from build123d import *

# Parameters (mm, degrees)
SKETCH3_OUTSIDE_W  = 93.666
SKETCH3_OUTSIDE_H  = 93.666
SKETCH3_OUTSIDE_R  = 6.5
CUT_EXTRUDE1_DEPTH = 21
SKETCH4_W          = 2.5
SKETCH4_H          = 24.819260196
SKETCH7_W          = 2.358889098
SKETCH7_H          = 15
CUT_EXTRUDE2_DEPTH = 12
CIRPATTERN1_COUNT  = 2
CIRPATTERN1_ANGLE  = 180
CHAMFER1_SIZE      = 0.5


with BuildPart() as part:
    # Sketch1 → Revolve1 (revolve)
    with BuildSketch(Plane(origin=(0, 0, 0), x_dir=(0, 0, -1), z_dir=(1, 0, 0)), mode=Mode.PRIVATE) as revolve1_sk:
        Polygon((14, 13), (0.5, 13), (0, 12.5), (0, 7.95), (2, 5.95), (19, 5.95), (20.171678207, 4), (38, 4), (40.403442476, 0), (44, 0), (44, 9.45), (43.5, 9.95), (41.5, 9.95), (41.5, 8.15), (38.3, 8.15), (38.3, 9.95), (35.8, 9.95), (35.8, 8.15), (30.8, 8.15), (30.8, 9.95), (28.3, 9.95), (28.3, 8.15), (25.1, 8.15), (25.1, 9.95), (21, 9.95), (21, 35), (14, 35), align=None)
    revolve(revolve1_sk.sketch.rotate(Axis((0, 0, 0), (0, 0, -1)), 90), axis=Axis((0, 0, 0), (0, 0, -1)))

    # Sketch3 outside → Cut-Extrude1 (cut)
    # profile 1 of 3: a face of its own
    with BuildSketch(Plane.XY):
        Rectangle(SKETCH3_OUTSIDE_W, SKETCH3_OUTSIDE_H)
        with BuildLine():
            Line((-20, 11.295529415), (-20, -11.295529415))
            ThreePointArc((-20, -11.295529415), (-19.765527652, -13.448311261), (-19.073106065, -15.500139543))
            Line((-19.073106065, -15.500139543), (-13.185668477, -28.204610128))
            ThreePointArc((-13.185668477, -28.204610128), (-9.495586596, -32.427517466), (-4.112562412, -34))
            Line((-4.112562412, -34), (4.112562412, -34))
            ThreePointArc((4.112562412, -34), (9.495586596, -32.427517466), (13.185668477, -28.204610128))
            Line((13.185668477, -28.204610128), (19.073106065, -15.500139543))
            ThreePointArc((19.073106065, -15.500139543), (19.765527652, -13.448311261), (20, -11.295529415))
            Line((20, -11.295529415), (20, 11.295529415))
            ThreePointArc((20, 11.295529415), (19.765527652, 13.448311261), (19.073106065, 15.500139543))
            Line((19.073106065, 15.500139543), (13.185668477, 28.204610128))
            ThreePointArc((13.185668477, 28.204610128), (9.495586596, 32.427517466), (4.112562412, 34))
            Line((4.112562412, 34), (-4.112562412, 34))
            ThreePointArc((-4.112562412, 34), (-9.495586596, 32.427517466), (-13.185668477, 28.204610128))
            Line((-13.185668477, 28.204610128), (-19.073106065, 15.500139543))
            ThreePointArc((-19.073106065, 15.500139543), (-19.765527652, 13.448311261), (-20, 11.295529415))
        make_face(mode=Mode.SUBTRACT)
    # profile 2 of 3: a face of its own
    with BuildSketch(Plane.XY):
        with Locations((0, 24)):
            Circle(SKETCH3_OUTSIDE_R)
    # profile 3 of 3: a face of its own
    with BuildSketch(Plane.XY):
        with Locations((0, -24)):
            Circle(SKETCH3_OUTSIDE_R)
    extrude(amount=-CUT_EXTRUDE1_DEPTH, mode=Mode.SUBTRACT)

    # Sketch4 → Cut-Revolve1 (revolve, cut)
    with BuildSketch(Plane(origin=(0, 0, 0), x_dir=(0, 0, -1), z_dir=(1, 0, 0)), mode=Mode.PRIVATE) as cut_revolve1_sk:
        with Locations((34.55, 0)):
            Rectangle(SKETCH4_W, SKETCH4_H)
    revolve(cut_revolve1_sk.sketch.rotate(Axis((0, 12.409630098, -33.3), (0, -1, 0)), 180), axis=Axis((0, 12.409630098, -33.3), (0, -1, 0)), mode=Mode.SUBTRACT)

    # Sketch7 → Cut-Extrude2 (cut)
    with BuildSketch(Plane.XY):
        with Locations((-13.179444549, -0.815585695)):
            Rectangle(SKETCH7_W, SKETCH7_H)
    cut_extrude2 = extrude(amount=-CUT_EXTRUDE2_DEPTH, mode=Mode.SUBTRACT)

    # CirPattern1: Cut-Extrude2 ×2 about axis
    cirpattern1_axis = Axis((0, 0, 0), (0, 0, 1))
    for i in range(1, CIRPATTERN1_COUNT):
        add(cut_extrude2.rotate(cirpattern1_axis, i * CIRPATTERN1_ANGLE / (CIRPATTERN1_COUNT - 1)), mode=Mode.SUBTRACT)

    # Chamfer1
    chamfer1_edges = [part.edges().sort_by_distance(p)[0] for p in [
        (-6.5, 24, -21),
        (-6.5, 24, -14),
        (-6.5, -24, -21),
        (-6.5, -24, -14),
        (0, 34, -21),
        (-9.495586596, 32.427517466, -21),
        (-16.129387271, 21.852374836, -21),
        (-19.765527652, 13.448311261, -21),
        (-20, 0, -21),
        (-19.765527652, -13.448311261, -21),
        (-16.129387271, -21.852374836, -21),
        (-9.495586596, -32.427517466, -21),
        (0, -34, -21),
        (9.495586596, -32.427517466, -21),
        (16.129387271, -21.852374836, -21),
        (19.765527652, -13.448311261, -21),
        (20, 0, -21),
        (19.765527652, 13.448311261, -21),
        (16.129387271, 21.852374836, -21),
        (9.495586596, 32.427517466, -21),
        (-9.495586596, 32.427517466, -14),
        (0, 34, -14),
        (9.495586596, 32.427517466, -14),
        (16.129387271, 21.852374836, -14),
        (19.765527652, 13.448311261, -14),
        (20, 0, -14),
        (19.765527652, -13.448311261, -14),
        (16.129387271, -21.852374836, -14),
        (9.495586596, -32.427517466, -14),
        (0, -34, -14),
        (-9.495586596, -32.427517466, -14),
        (-16.129387271, -21.852374836, -14),
        (-19.765527652, -13.448311261, -14),
        (-20, 0, -14),
        (-19.765527652, 13.448311261, -14),
        (-16.129387271, 21.852374836, -14),
    ]]
    chamfer(chamfer1_edges, length=CHAMFER1_SIZE)


solid = part.part
CAD build for the part. Positions are in the model's coordinates, mm. A direction names the side the tool comes from. Round coordinates to 2 decimals unless told otherwise and drop trailing zeros. Loops run counter-clockwise (first coordinate to the right, second up) from the corner with the lowest first, then second, coordinate; pieces in that order, holes last. Notation, with made-up numbers: (81, -15.5) - (115, -15.5) arc R10 cw to (115, 1.5) - close; hole circle Ø4 at (72, 49.5). An arc over 180 degrees is marked (long way). Put each result on its own line as item: value.
1. Slice it at C-C on y = -24. List the corners of the cut face in (x, z), and give its area (3 significant figures).
Geometry check:
outline: (-15.13, -20.5) - (-14.58, -21) - (-7, -21) - (-6.5, -20.5) - (-6.5, -14.5) - (-7, -14) - (-14.58, -14) - (-15.13, -14.5) - close; (6.5, -20.5) - (7, -21) - (14.58, -21) - (15.13, -20.5) - (15.13, -14.5) - (14.58, -14) - (7, -14) - (6.5, -14.5) - close
area: 120 mm²
2. Two-plate mould, pull along Z, no slides. Class faces 1 (the conical face through (-9.235, 32.161, -20.865)), 2 (the flat face through (0, 34, -17)), 3 (the flat face through (-15.86, 21.84, -14.25)), 4 (the flat face through (-8.2, -1.5, -28.3)): released by +Z, released by -Z, zero draft, split by the parting line, or undercut.
Geometry check:
face 1: released by -Z
face 2: zero draft
face 3: released by +Z
face 4: undercut
3. Pin check, flat tips, straight feed: P1, Ø21, axis at x = 0, y = -24, coming from the +Z side; P2, Ø4, axis at x = -8.5, z = -20.5, coming from the +Y side; P3, Ø8, axis at x = 13.5, z = -8, coming from the +Y side; P4, Ø1, axis at x = -9.5, z = -26.5, coming from the +Y side. Stop position of each tip, or through.
Geometry check:
P1: z = -14
P2: y = 33.71
P3: y = 8.87
P4: through
4. 3-axis set-ups, long thin cutter, end or side, ignore diameter. For faces 5 (the cylindrical face through (-7.9, 6.05, -29.53)), 6 (the cylindrical face through (-4.385, -4.021, -10.619)), 7 (the flat face through (8.2, -1.5, -25.1)): which of +Z, -Z, +X, -X, +Y, -Y reach the whole face in a straight line?
Geometry check:
face 5: -Z
face 6: +Z
face 7: none
5. Slice it at B-B on z = -5.5. List the corners of the cut face in (x, y), and give its area (3 significant figures).
Geometry check:
outline: (-12, -5) arc R13 ccw to (12, -5) - (12, 5) arc R13 ccw to (-12, 5) - close; hole circle Ø11.9 at (0, 0)
area: 406 mm²
6. Slice it at D-D on z = -33.3. List the corners of the cut face in (x, y), and give its area (3 significant figures).
Geometry check:
outline: (-2.5, -7.76) - (-2.5, -3.12) arc R4 cw to (-2.5, 3.12) - (-2.5, 7.76) arc R8.15 ccw to start; (2.5, -7.76) arc R8.15 ccw to (2.5, 7.76) - (2.5, 3.12) arc R4 cw to (2.5, -3.12) - close
area: 115 mm²
7. Slice it at A-A on z = -16.5. List the corners of the cut face in (x, y).
Geometry check:
outline: (-20, -11.3) arc R10 ccw to (-19.07, -15.5) - (-13.19, -28.2) arc R10 ccw to (-4.11, -34) - (4.11, -34) arc R10 ccw to (13.19, -28.2) - (19.07, -15.5) arc R10 ccw to (20, -11.3) - (20, 11.3) arc R10 ccw to (19.07, 15.5) - (13.19, 28.2) arc R10 ccw to (4.11, 34) - (-4.11, 34) arc R10 ccw to (-13.19, 28.2) - (-19.07, 15.5) arc R10 ccw to (-20, 11.3) - close; hole circle Ø13 at (0, -24); hole circle Ø13 at (0, 24); hole circle Ø11.9 at (0, 0)
8. Wall check: line 1 (Y direction, x = 0, z = -18); line 2 (Y direction, x = 0, z = -6); line 3 (Z direction, x = -15.5, y = 5). Give the ranges that are in metal, low to high.
Geometry check:
line 1: -34 to -30.5, -17.5 to -5.95, 5.95 to 17.5, 30.5 to 34
line 2: -13 to -5.95, 5.95 to 13
line 3: -21 to -14
